```python
from build123d import *

# Parameters (mm, degrees)
SKETCH1_R                                  = 3.175
BOSS_EXTRUDE1_DEPTH                        = 3.556
SKETCH2_R                                  = 0.79375
CUT_EXTRUDE1_DEPTH                         = 4.556
SKETCH3_R                                  = 0.79375
CUT_EXTRUDE2_DEPTH                         = 3.175
SKETCH4_W                                  = 0.79375
SKETCH4_H                                  = 4.469902345
CUT_EXTRUDE3_DEPTH                         = 4.556
SKETCH5_R                                  = 1.5875
CUT_EXTRUDE4_DEPTH                         = 1.778
MIRROR1_AT_THE_SECOND_PLANE_COPY_1_SKETC_R = 1.5875
MIRROR1_AT_THE_SECOND_PLANE_COPY_1_DEPTH   = 1.778


with BuildPart() as part:
    # Sketch1 → Boss-Extrude1 (new body)
    with BuildSketch(Plane(origin=(0, 0, 0), x_dir=(1, 0, 0), z_dir=(0, 1, 0))):
        Polygon((-1.5875, 7.62), (-1.5875, 10.922), (-0.396875, 10.922), (-0.396875, 7.62), (0.396875, 7.62), (0.396875, 10.922), (1.5875, 10.922), (1.5875, 7.62), (7.62, 7.62), (7.62, -7.62), (-7.62, -7.62), (-7.62, 7.62), align=None)
        Circle(SKETCH1_R, mode=Mode.SUBTRACT)
    extrude(amount=BOSS_EXTRUDE1_DEPTH)

    # Sketch2 → Cut-Extrude1 (cut, through all)
    with BuildSketch(Plane(origin=(0, 3.556, 0), x_dir=(1, 0, 0), z_dir=(0, 1, 0))):
        with Locations((-4.939140867, 4.939140867)):
            Circle(SKETCH2_R)
        with Locations((4.939140867, 4.939140867)):
            Circle(SKETCH2_R)
        with Locations((4.939140867, -4.939140867)):
            Circle(SKETCH2_R)
        with Locations((-4.939140867, -4.939140867)):
            Circle(SKETCH2_R)
    extrude(amount=-CUT_EXTRUDE1_DEPTH, mode=Mode.SUBTRACT)

    # Sketch3 → Cut-Extrude2 (cut)
    with BuildSketch(Plane(origin=(1.5875, 0, 0), x_dir=(0, 0, -1), z_dir=(1, 0, 0))):
        with Locations((9.271, 1.778)):
            Circle(SKETCH3_R)
    extrude(amount=-CUT_EXTRUDE2_DEPTH, mode=Mode.SUBTRACT)

    # Sketch4 → Cut-Extrude3 (cut, through all)
    with BuildSketch(Plane(origin=(0, 3.556, 0), x_dir=(1, 0, 0), z_dir=(0, 1, 0))):
        with Locations((0, 5.385048828)):
            Rectangle(SKETCH4_W, SKETCH4_H)
    extrude(amount=-CUT_EXTRUDE3_DEPTH, mode=Mode.SUBTRACT)

    # Sketch5 → Cut-Extrude4 (cut)
    with BuildSketch(Plane(origin=(0, 3.556, 0), x_dir=(1, 0, 0), z_dir=(0, 1, 0))):
        with Locations((-4.939140867, 4.939140867)):
            Circle(SKETCH5_R)
    cut_extrude4 = extrude(amount=-CUT_EXTRUDE4_DEPTH, mode=Mode.SUBTRACT)

    # Mirror1: Cut-Extrude4 across plane
    add(cut_extrude4.mirror(Plane.XY), mode=Mode.SUBTRACT)

    # Mirror1 at the second plane: Cut-Extrude4 across plane
    add(cut_extrude4.mirror(Plane(origin=(0, 0, 0), x_dir=(0, 0, 1), z_dir=(1, 0, 0))), mode=Mode.SUBTRACT)

    # Mirror1 at the second plane copy 1 sketc → Mirror1 at the second plane copy 1 (cut)
    with BuildSketch(Plane(origin=(0, 3.556, 0), x_dir=(-1, 0, 0), z_dir=(0, 1, 0))):
        with Locations((-4.939140867, 4.939140867)):
            Circle(MIRROR1_AT_THE_SECOND_PLANE_COPY_1_SKETC_R)
    extrude(amount=-MIRROR1_AT_THE_SECOND_PLANE_COPY_1_DEPTH, mode=Mode.SUBTRACT)


solid = part.part
```
Read the model definition and answer for the solid it produces. Units are mm, in the model's axes. A direction names the side the tool comes from. Give positions to 0.01 mm unless a question says otherwise; leave off trailing zeros. Order: outer loops, then holes, each group sorted by start corner. A loop starts at its lowest first (then second) coordinate and runs counter-clockwise, first axis right, second up. Notation, with made-up numbers: (14, -8.5) -> (49, -8.5) arc R25 ccw to (49, 11.5) -> close; hole circle Ø2 at (80.25, -33). An arc over 180 degrees is marked (long way). Write item = value, one per line.
1. A cutting plane is placed at C-C, the plane y = 1.4. Count the separate pieces of the cut face and the enclosed holes in it, and give its area (3 significant figures).
Numbers:
separate_pieces = 3
enclosed_holes = 4
area = 194 mm²
2. A cutting plane is placed at B-B, the plane x = 5.25. Write down the section's boundary in (y, z).
Numbers:
outline = (0, -7.62) -> (3.56, -7.62) -> (3.56, -6.5) -> (1.78, -6.5) -> (1.78, -5.67) -> (0, -5.67) -> close; (0, -4.21) -> (1.78, -4.21) -> (1.78, -3.38) -> (3.56, -3.38) -> (3.56, 3.38) -> (1.78, 3.38) -> (1.78, 4.21) -> (0, 4.21) -> close; (0, 5.67) -> (1.78, 5.67) -> (1.78, 6.5) -> (3.56, 6.5) -> (3.56, 7.62) -> (0, 7.62) -> close
3. Given pin 1 (2.5 mm diameter, centred on x = 4.94, z = -4.94, fed in from +Y); pin 2 (1.8 mm diameter, centred on x = -4.5, y = 2.5, fed in from -Z), each flat-ended and moving along its own axis, determine where each tip first touches the part or whether it passes through.
Numbers:
pin_1 = 1.78
pin_2 = -7.62
4. The mould has two halves that part along X. Classify faces 1 (the face through (1.588, 1, -10)), 2 (the face through (-6.11, 2.68, -6.01)), 3 (the face through (-1, 2, -10.922)), 4 (the face through (-6, 1.778, 5)): +X half, -X half, draft (parallel to the pull), parting line (faces both ways), or undercut.
Numbers:
face_1 = +X half
face_2 = undercut
face_3 = draft
face_4 = undercut
5. For faces 5 (the face through (0.397, 2, -7)), 6 (the face through (6, 1.778, 5)), 7 (the face through (-5, 2, -7.62)), determine the directions among +Z, -Z, +X, -X, +Y, -Y from which every point of the face is accessible in a straight line to the end or side of a thin tool.
Numbers:
face_5 = -Z, +Y, -Y
face_6 = +Y
face_7 = -Z, -X, +Y, -Y
6. Straight lines are drawn through the part: line 1 along X through (y, z) = (1.2, 5); line 2 along Z through (x, y) = (-2.75, 0.65); line 3 along X through (y, z) = (1.4, -7.25). For each, find the intervals that lie inside material, in ascending order.
Numbers:
line_1 = -7.62 to -5.73, -4.15 to 4.15, 5.73 to 7.62
line_2 = -7.62 to -1.59, 1.59 to 7.62
line_3 = -7.62 to -0.4, 0.4 to 7.62
7. A cutting plane is placed at D-D, the plane z = -8.75. Write down the section's boundary in (x, y).
Numbers:
outline = (-1.59, 0) -> (-0.4, 0) -> (-0.4, 1.18) -> (-1.59, 1.18) -> close; (-1.59, 2.38) -> (-0.4, 2.38) -> (-0.4, 3.56) -> (-1.59, 3.56) -> close; (0.4, 0) -> (1.59, 0) -> (1.59, 1.18) -> (0.4, 1.18) -> close; (0.4, 2.38) -> (1.59, 2.38) -> (1.59, 3.56) -> (0.4, 3.56) -> close
8. A cutting plane is placed at A-A, the plane z = 0. Write down the section's boundary in (x, y) (3 decimals), and give its area (3 significant figures).
Numbers:
outline = (-7.62, 0) -> (-3.175, 0) -> (-3.175, 3.556) -> (-7.62, 3.556) -> close; (3.175, 0) -> (7.62, 0) -> (7.62, 3.556) -> (3.175, 3.556) -> close
area = 31.6 mm²
